Read the model definition and answer for the solid it produces. Units are mm, in the model's axes. Face numbers are marked on the shaded views. A direction names the side the tool comes from. Round coordinates to 2 decimals unless told otherwise and drop trailing zeros. Order: outer loops, then holes, each group sorted by start corner. A loop starts at its lowest first (then second) coordinate and runs counter-clockwise, first axis right, second up.
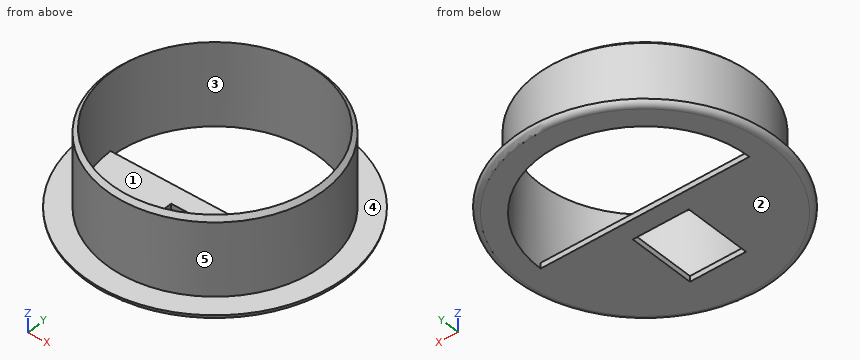
from build123d import *

# Parameters (mm, degrees)
F0_R     = 46.75
F0_R_2   = 38.75
F1_DEPTH = 2
F0_W     = 20
F0_H     = 24
F2_DEPTH = 30
F4_R     = 1.99999


# Not quite as in the source:
# - a fillet or chamfer that OpenCascade refuses, or shapes differently, is made with other operations: its cross-section is extruded or revolved along the edge and cut away or added
# - a fillet or chamfer is up to 0.001 mm smaller than in the source, because OpenCascade refuses the exact size


with BuildPart() as f1:
    # F0 (on Top) → F1 (new body)
    with BuildSketch(Plane.XY):
        Circle(F0_R)
        Circle(F0_R_2, mode=Mode.SUBTRACT)
    extrude(amount=F1_DEPTH)



with BuildPart() as f1b:
    # F0 (on Top) → F1, piece 2 (new body)
    with BuildSketch(Plane.XY):
        with BuildLine():
            ThreePointArc((-37.25, 0), (0, -37.25), (37.25, 0))
            Line((37.25, 0), (-37.25, 0))
        make_face()
        with Locations((0, -18.625)):
            Rectangle(F0_W, F0_H, mode=Mode.SUBTRACT)
    extrude(amount=F1_DEPTH)


with BuildPart() as f1_1:
    add(f1.part)

    add(f1b.part)  # F2 merges F1b
    # F0 (on Top) → F2 (join)
    with BuildSketch(Plane.XY):
        Circle(F0_R_2)
        with BuildLine():
            ThreePointArc((-37.25, 0), (0, 37.25), (37.25, 0))
            ThreePointArc((37.25, 0), (0, -37.25), (-37.25, 0))
        make_face(mode=Mode.SUBTRACT)
    extrude(amount=F2_DEPTH)

    # F3: chamfer of 2 on 1 edges, made by hand

    # F3_s1 → F3_t2 (revolve, cut)
    with BuildSketch(Plane.XZ):
        Polygon((36.75, 30), (38.75, 28), (38.75, 30), align=None)
    revolve(axis=Axis((0, 0, 30), (0, 0, 1)), mode=Mode.SUBTRACT)

    # F4 (radius 2 in the source; OpenCascade refuses exactly that, so slightly less here)
    f4_edges = [f1_1.edges().sort_by_distance(p)[0] for p in [
        (-46.75, 0, 0),
    ]]
    fillet(f4_edges, radius=F4_R)


solid = f1_1.part
Q1. For the marked faces 1 and 2, determine the directions among +Z, -Z, +X, -X, +Y, -Y from which every point of the face is accessible in a straight line to the end or side of a thin tool.
Outcome:
face 1: +Z
face 2: -Z, +X, -X, +Y, -Y
Q2. Straight lines are drawn through the part: probe 1 along Y at (x, z) = (0, 18.25); probe 2 along Y at (x, z) = (-17.5, 6); probe 3 along X at (y, z) = (34, 26.75). For each, find the intervals that lie inside material, in ascending order.
Outcome:
probe 1: y = -38.75 to -37.25, 37.25 to 38.75
probe 2: y = -34.57 to -32.88, 32.88 to 34.57
probe 3: x = -18.59 to -15.22, 15.22 to 18.59
Q3. For a pull along X with two mould halves and no side action, classify the marked faces 3, 4 and 5 as released by +X, released by -X, zero draft, split by the parting line, or undercut.
Outcome:
face 3: undercut
face 4: zero draft
face 5: split by the parting line
Q4. Flat-ended cylindrical pins translate along their axes: pin 1 (1 mm diameter, centred on y = -3, z = 15.5, fed in from -X); pin 2 (1 mm diameter, centred on x = 0.5, z = 0.5, fed in from -Y); pin 3 (1 mm diameter, centred on y = -15.5, z = 0.5, fed in from -X). Find the tip coordinate at first contact, or state that the pin passes through.
Outcome:
pin 1: stops at x = -38.67
pin 2: stops at y = -46.48
pin 3: stops at x = -43.87
Q5. A cutting plane is placed at B-B, the plane z = 26.5. Give the vertices of the cut face in (x, y), plus the area to 3 significant figures.
Outcome:
outline: circle Ø77.5 at (0, 0); hole circle Ø74.5 at (0, 0)
area: 358 mm2
Q6. A cutting plane is placed at A-A, the plane x = 0. Give the number of separate pieces and of enclosed holes in the cut face, plus the area to 3 significant figures.
Outcome:
separate pieces: 3
enclosed holes: 0
area: 143 mm2
